```python
from build123d import *

# Parameters (mm, degrees)
SKETCH1_R           = 10
BOSS_EXTRUDE1_DEPTH = 150
BOSS_EXTRUDE2_DEPTH = 5
CHAMFER1_SIZE       = 1
CHAMFER3_SIZE       = 2.5


with BuildPart() as part:
    # Sketch1 → Boss-Extrude1 (new body)
    with BuildSketch(Plane(origin=(0, 0, 0), x_dir=(0, 0, -1), z_dir=(1, 0, 0))):
        Circle(SKETCH1_R)
    extrude(amount=BOSS_EXTRUDE1_DEPTH)

    # Sketch2 → Boss-Extrude2 (add)
    with BuildSketch(Plane(origin=(150, 0, 0), x_dir=(0, 0, -1), z_dir=(1, 0, 0))):
        Polygon((-16.308454096, 0.29661326), (-8.411101666, -13.975228914), (7.89735243, -14.271842174), (16.308454096, -0.29661326), (8.411101666, 13.975228914), (-7.89735243, 14.271842174), align=None)
    extrude(amount=BOSS_EXTRUDE2_DEPTH)

    # Chamfer1
    chamfer1_edges = [part.edges().sort_by_distance(p)[0] for p in [
        (155, 7.284227717, 12.102903263),
        (155, -6.839307827, 12.359777881),
        (155, -14.123535544, 0.256874618),
        (155, -7.284227717, -12.102903263),
        (155, 6.839307827, -12.359777881),
        (155, 14.123535544, -0.256874618),
    ]]
    chamfer(chamfer1_edges, length=CHAMFER1_SIZE)

    # Chamfer3
    chamfer3_edges = [part.edges().sort_by_distance(p)[0] for p in [
        (0, 0, 10),
    ]]
    chamfer(chamfer3_edges, length=CHAMFER3_SIZE)


solid = part.part
```
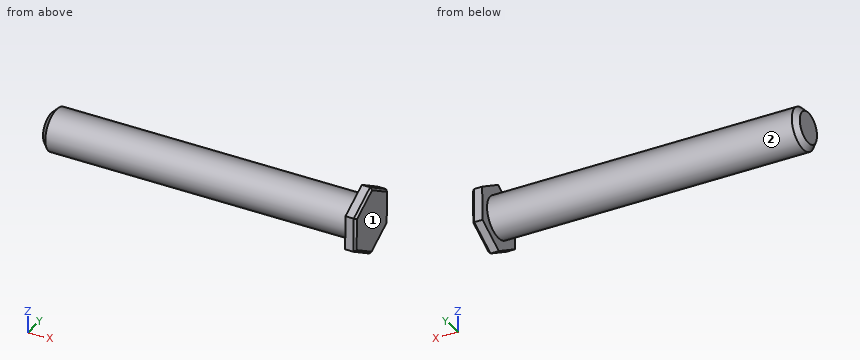
Can you work these out from the model? Positions are in its coordinate system, mm. Face numbers are marked on the shaded views. A direction names the side the tool comes from. Round coordinates to 2 decimals unless told otherwise and drop trailing zeros. Loops run counter-clockwise (first coordinate to the right, second up) from the corner with the lowest first, then second, coordinate; pieces in that order, holes last. Notation, with made-up numbers: M 70.5,58 L 103.5,58 A17 ccw 103.5,81 Z; hole C 81.25,-9 d7. An arc over 180 degrees is marked long. Answer as a JSON object with one key per item and string values. Group by question number.
Q1. Will these pins go through, and if not, where does the flat tip stop? pin 1 (3 mm diameter, centred on x = 45.5, z = 1.5, fed in from -Y); pin 2 (12 mm diameter, centred on x = 72.5, z = -10.5, fed in from +Y); pin 3 (3 mm diameter, centred on x = 136, y = -3, fed in from -Z).
Q2. On a 3-axis mill with a long thin cutter (end or side, diameter ignored), from which of +Z, -Z, +X, -X, +Y, -Y can I reach the whole of each face in a straight line? I mean the marked faces 1 and 2. Say none if no direction works.
Q3. Imagine slicing it at B-B, the plane z = 0. Please give me the cut outline in (x, y), then the cut area to 3 significant figures.
Q4. Imagine slicing it at C-C, the plane z = 13.5. Please give me the cut outline in (x, y).
Q5. Please list where these lines run through material, in increasing order: L1, parallel to X at y = 12.75, z = -0.5; L2, parallel to Z at x = 96, y = 0.5; L3, parallel to Z at x = 74.5, y = -4.25.
Q6. Imagine slicing it at A-A, the plane x = 118. Please give me the cut outline in (y, z).
Findings:
{
 "1": {"pin 1": "stops at y = -10", "pin 2": "stops at y = 8.93", "pin 3": "stops at z = -9.89"},
 "2": {"face 1": "+Z, -Z, +X, +Y, -Y", "face 2": "-X"},
 "3": {"outline": "M 0,-7.5 L 2.5,-10 L 150,-10 L 150,-14.13 L 154,-14.13 L 155,-13.13 L 155,13.13 L 154,14.13 L 150,14.13 L 150,10 L 2.5,10 L 0,7.5 Z", "area": "3,130 mm2"},
 "4": {"outline": "M 150,-4.78 L 154,-4.78 L 155,-2.71 L 155,3.02 L 154,4.96 L 150,4.96 Z"},
 "5": {"L1": "x = 150 to 155", "L2": "z = -9.99 to 9.99", "L3": "z = -9.05 to 9.05"},
 "6": {"outline": "C 0,0 d20"}
}
